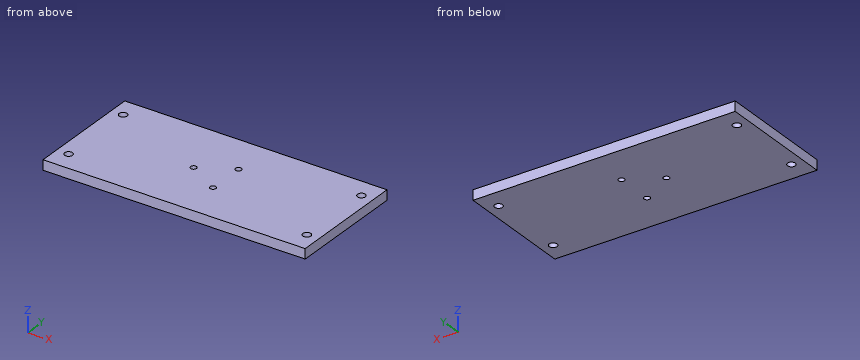
```python
from build123d import *

# Parameters (mm, degrees)
SKETCH1_W           = 140
SKETCH1_H           = 60
BOSS_EXTRUDE1_DEPTH = 5
CUT_EXTRUDE1_REACH  = 7
SKETCH2_R           = 2
SKETCH3_W           = 4
SKETCH3_H           = 60
CUT_EXTRUDE2_DEPTH  = 6
CUT_EXTRUDE3_REACH  = 7
SKETCH4_R           = 1.5


with BuildPart() as part:
    # Sketch1 → Boss-Extrude1 (new body)
    with BuildSketch(Plane.XY):
        Rectangle(SKETCH1_W, SKETCH1_H)
    extrude(amount=BOSS_EXTRUDE1_DEPTH)

    # Sketch2 → Cut-Extrude1 (cut, up to next)
    with BuildSketch(Plane.XY.offset(5), mode=Mode.PRIVATE) as cut_extrude1_sk1:
        with Locations((-60, 20)):
            Circle(SKETCH2_R)
    cut_extrude1_tool1 = extrude(cut_extrude1_sk1.sketch, amount=-CUT_EXTRUDE1_REACH, mode=Mode.PRIVATE) & part.part
    add(cut_extrude1_tool1.solids().sort_by_distance((-60, 20, 5))[0], mode=Mode.SUBTRACT)
    # Sketch2 → Cut-Extrude1 (cut, up to next)
    with BuildSketch(Plane.XY.offset(5), mode=Mode.PRIVATE) as cut_extrude1_sk2:
        with Locations((60, 20)):
            Circle(SKETCH2_R)
    cut_extrude1_tool2 = extrude(cut_extrude1_sk2.sketch, amount=-CUT_EXTRUDE1_REACH, mode=Mode.PRIVATE) & part.part
    add(cut_extrude1_tool2.solids().sort_by_distance((60, 20, 5))[0], mode=Mode.SUBTRACT)
    # Sketch2 → Cut-Extrude1 (cut, up to next)
    with BuildSketch(Plane.XY.offset(5), mode=Mode.PRIVATE) as cut_extrude1_sk3:
        with Locations((60, -20)):
            Circle(SKETCH2_R)
    cut_extrude1_tool3 = extrude(cut_extrude1_sk3.sketch, amount=-CUT_EXTRUDE1_REACH, mode=Mode.PRIVATE) & part.part
    add(cut_extrude1_tool3.solids().sort_by_distance((60, -20, 5))[0], mode=Mode.SUBTRACT)
    # Sketch2 → Cut-Extrude1 (cut, up to next)
    with BuildSketch(Plane.XY.offset(5), mode=Mode.PRIVATE) as cut_extrude1_sk4:
        with Locations((-60, -20)):
            Circle(SKETCH2_R)
    cut_extrude1_tool4 = extrude(cut_extrude1_sk4.sketch, amount=-CUT_EXTRUDE1_REACH, mode=Mode.PRIVATE) & part.part
    add(cut_extrude1_tool4.solids().sort_by_distance((-60, -20, 5))[0], mode=Mode.SUBTRACT)

    # Sketch3 → Cut-Extrude2 (cut, through all)
    with BuildSketch(Plane.XY.offset(5)):
        with Locations((-68, 0)):
            Rectangle(SKETCH3_W, SKETCH3_H)
        with Locations((68, 0)):
            Rectangle(SKETCH3_W, SKETCH3_H)
    extrude(amount=-CUT_EXTRUDE2_DEPTH, mode=Mode.SUBTRACT)

    # Sketch4 → Cut-Extrude3 (cut, up to next)
    with BuildSketch(Plane.XY.offset(5), mode=Mode.PRIVATE) as cut_extrude3_sk1:
        with Locations((5.3975, 9.348744234)):
            Circle(SKETCH4_R)
    cut_extrude3_tool1 = extrude(cut_extrude3_sk1.sketch, amount=-CUT_EXTRUDE3_REACH, mode=Mode.PRIVATE) & part.part
    add(cut_extrude3_tool1.solids().sort_by_distance((5.3975, 9.348744, 5))[0], mode=Mode.SUBTRACT)
    # Sketch4 → Cut-Extrude3 (cut, up to next)
    with BuildSketch(Plane.XY.offset(5), mode=Mode.PRIVATE) as cut_extrude3_sk2:
        with Locations((5.3975, -9.348744234)):
            Circle(SKETCH4_R)
    cut_extrude3_tool2 = extrude(cut_extrude3_sk2.sketch, amount=-CUT_EXTRUDE3_REACH, mode=Mode.PRIVATE) & part.part
    add(cut_extrude3_tool2.solids().sort_by_distance((5.3975, -9.348744, 5))[0], mode=Mode.SUBTRACT)
    # Sketch4 → Cut-Extrude3 (cut, up to next)
    with BuildSketch(Plane.XY.offset(5), mode=Mode.PRIVATE) as cut_extrude3_sk3:
        with Locations((-10.795, 0)):
            Circle(SKETCH4_R)
    cut_extrude3_tool3 = extrude(cut_extrude3_sk3.sketch, amount=-CUT_EXTRUDE3_REACH, mode=Mode.PRIVATE) & part.part
    add(cut_extrude3_tool3.solids().sort_by_distance((-10.795, 0, 5))[0], mode=Mode.SUBTRACT)


solid = part.part
```
The listing builds one solid part. Answer for the finished solid, in the listing's coordinates (mm). Give positions to 0.01 mm unless a question says otherwise; leave off trailing zeros. Order: outer loops, then holes, each group sorted by start corner. A loop starts at its lowest first (then second) coordinate and runs counter-clockwise, first axis right, second up. Notation, with made-up numbers: (10.25, 27.25) -> (15.25, 27.25) arc R27 cw to (15.25, 49.25) -> close; hole circle Ø4 at (62, -30.75). An arc over 180 degrees is marked (long way). Answer as CSV lines item,"result". Start each with the question number.
Q1. A cutting plane is placed at A-A (y = 20). Determine the outline of the cut face in (x, z), then the cut area to 3 significant figures.
Q2. A cutting plane is placed at C-C (y = 0). Determine the outline of the cut face in (x, z) (3 decimals).
Q3. A cutting plane is placed at B-B (x = 60). Determine the outline of the cut face in (y, z), then the cut area to 3 significant figures.
Q4. Find the intervals of material crossed by L1, parallel to Y at x = -60, z = 3; L2, parallel to X at y = -9.5, z = 2.5; L3, parallel to X at y = 20.5, z = 3.25, in increasing order.
Results found:
1,outline,"(-66, 0) -> (-62, 0) -> (-62, 5) -> (-66, 5) -> close; (-58, 0) -> (58, 0) -> (58, 5) -> (-58, 5) -> close; (62, 0) -> (66, 0) -> (66, 5) -> (62, 5) -> close"
1,area,"620 mm2"
2,outline,"(-66, 0) -> (-12.295, 0) -> (-12.295, 5) -> (-66, 5) -> close; (-9.295, 0) -> (66, 0) -> (66, 5) -> (-9.295, 5) -> close"
3,outline,"(-30, 0) -> (-22, 0) -> (-22, 5) -> (-30, 5) -> close; (-18, 0) -> (18, 0) -> (18, 5) -> (-18, 5) -> close; (22, 0) -> (30, 0) -> (30, 5) -> (22, 5) -> close"
3,area,"260 mm2"
4,L1,"-30 to -22, -18 to 18, 22 to 30"
4,L2,"-66 to 3.91, 6.89 to 66"
4,L3,"-66 to -61.94, -58.06 to 58.06, 61.94 to 66"
